from build123d import *

# Parameters (mm, degrees)
F0_R           = 1.7
F1_DEPTH       = 5
F3_D           = 3.4
F3_CSINK_D     = 6.72
F3_CSINK_ANGLE = 90


with BuildPart() as f1:
    # F0 (on Top) → F1 (new body)
    with BuildSketch(Plane.XY):
        Polygon((95, 13), (-95, 13), (-95, -13), (-85, -13), (-85, 11), (-30, 11), (-30, 3), (-30, -13), (-10, -13), (-10, 11), (45, 11), (45, 3), (45, -13), (65, -13), (65, 11), (95, 11), align=None)
        with Locations((-20, -7)):
            Circle(F0_R, mode=Mode.SUBTRACT)
        with Locations((55, -7)):
            Circle(F0_R, mode=Mode.SUBTRACT)
        with Locations((-20, 3)):
            Circle(F0_R, mode=Mode.SUBTRACT)
        with Locations((55, 3)):
            Circle(F0_R, mode=Mode.SUBTRACT)
    extrude(amount=F1_DEPTH)

    # F3 (through all)
    with Locations(Plane.XY.offset(5)):
        with Locations((-20, 3), (-20, -7), (55, 3), (55, -7)):
            CounterSinkHole(F3_D / 2, F3_CSINK_D / 2, counter_sink_angle=F3_CSINK_ANGLE)


solid = f1.part
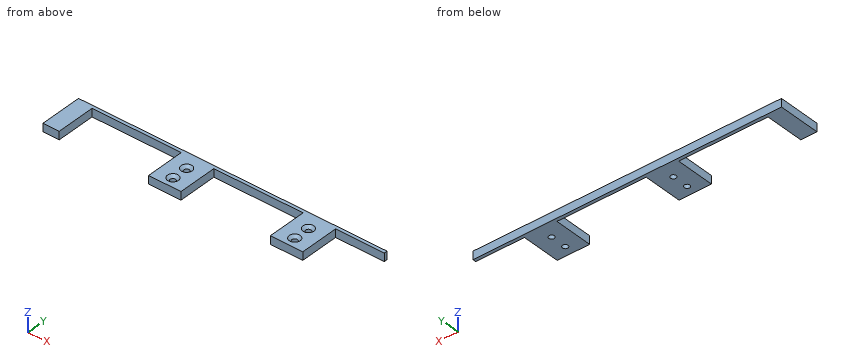
Verification items for the finished model (mm, model axes). Give positions to 0.01 mm unless a question says otherwise; leave off trailing zeros. Write each loop counter-clockwise with the first axis right and the second up, starting at its lowest first coordinate (ties: lowest second). Pieces come first, ordered by that corner, then holes.
(1) Cross-section at A-A (y = 8.75). Enter the section's corners in (x, z).
(2) Cross-section at B-B (y = -7). Enter the section's corners in (x, z), plus the area to 3 significant figures.
(3) Material ranges on line 1 (Y direction, x = 55, z = 0.8); line 2 (X direction, y = 1, z = 3.45); line 3 (X direction, y = 3, z = 2.6), recorded low to high.
(4) Gauge pin test, flat ends, axial feed: pin 1 (1.5 mm diameter, centred on y = 0, z = 3, fed in from +X); pin 2 (2 mm diameter, centred on x = 55, y = -7, fed in from +Z); pin 3 (1.5 mm diameter, centred on x = -50.5, z = 2, fed in from -Y). Record the tip position at first contact, or that the pin passes through.
(5) Cross-section at D-D (z = 2.2). Enter the section's corners in (x, y), plus the area to 3 significant figures.
(6) Cross-section at C-C (x = 55). Enter the section's corners in (y, z), plus the area to 3 significant figures.
Worked out:
1. outline: (-95, 0) - (-85, 0) - (-85, 5) - (-95, 5) - close; (-30, 0) - (-10, 0) - (-10, 5) - (-30, 5) - close; (45, 0) - (65, 0) - (65, 5) - (45, 5) - close
2. outline: (-95, 0) - (-85, 0) - (-85, 5) - (-95, 5) - close; (-30, 0) - (-21.7, 0) - (-21.7, 3.34) - (-23.36, 5) - (-30, 5) - close; (-18.3, 0) - (-10, 0) - (-10, 5) - (-16.64, 5) - (-18.3, 3.34) - close; (45, 0) - (53.3, 0) - (53.3, 3.34) - (51.64, 5) - (45, 5) - close; (56.7, 0) - (65, 0) - (65, 5) - (58.36, 5) - (56.7, 3.34) - close
2. area: 210 mm2
3. line 1: y = -13 to -8.7, -5.3 to 1.3, 4.7 to 13
3. line 2: x = -95 to -85, -30 to -10, 45 to 65
3. line 3: x = -95 to -85, -30 to -21.7, -18.3 to -10, 45 to 53.3, 56.7 to 65
4. pin 1: stops at x = 65
4. pin 2: passes through
4. pin 3: stops at y = 11
5. outline: (-95, -13) - (-85, -13) - (-85, 11) - (-30, 11) - (-30, -13) - (-10, -13) - (-10, 11) - (45, 11) - (45, -13) - (65, -13) - (65, 11) - (95, 11) - (95, 13) - (-95, 13) - close; hole circle Ø3.4 at (-20, -7); hole circle Ø3.4 at (-20, 3); hole circle Ø3.4 at (55, -7); hole circle Ø3.4 at (55, 3)
5. area: 1,540 mm2
6. outline: (-13, 0) - (-8.7, 0) - (-8.7, 3.34) - (-10.36, 5) - (-13, 5) - close; (-5.3, 0) - (1.3, 0) - (1.3, 3.34) - (-0.36, 5) - (-3.64, 5) - (-5.3, 3.34) - close; (4.7, 0) - (13, 0) - (13, 5) - (6.36, 5) - (4.7, 3.34) - close
6. area: 90.5 mm2
